The model under review builds one solid part; all positions refer to its coordinate system, in mm. Coordinates: 2 decimals unless noted, no trailing zeros. Write each loop counter-clockwise with the first axis right and the second up, starting at its lowest first coordinate (ties: lowest second). Pieces come first, ordered by that corner, then holes. Notation, with made-up numbers: (-25.75, -19) - (33.25, -19) arc R20 cw to (33.25, 0) - close; hole circle Ø5 at (-24, 76.25). An arc over 180 degrees is marked (long way). Return JSON: item names as keys, results as strings. Group by question number.
(1) We need section B-B on z = 159. State the section outline as (x, y) points, then the cut area to 3 significant figures.
(2) To check wall thickness, follow L1, parallel to X at y = -10, z = 160.5; L2, parallel to Z at x = 140.8, y = -4.75; L3, parallel to Z at x = 100.8, y = -5.5. State the ranges of each line that lie inside material, in increasing order. Write a range as from..to.
(3) We need section D-D on y = -6. State the section outline as (x, z) points (3 decimals).
(4) For pin 1 Ø11.5 at (x, z) = (180.8, 160) entering from +Y, flat-tipped, find the tip position at first contact; note if it passes through.
(5) We need section C-C on x = 140.8. State the section outline as (y, z) points.
(6) Draft analysis for pull direction X (two halves, no side actions). For faces 1 (the face through (90, -6, 145)), 2 (the face through (142, -12.7, 140)), 3 (the face through (100, -6.3, 166.3)), 4 (the face through (191.6, -6, 146)), state which applies: released by +X, released by -X, zero draft, split by the parting line, or undercut.
(7) We need section A-A on x = 100.8. State the section outline as (y, z) points, then the cut area to 3 significant figures.
```python
from build123d import *

# Parameters (mm, degrees)
SKETCH057_R  = 3.571875
PAD057_DEPTH = 30
SKETCH056_R  = 6.35
PAD056_DEPTH = 12.7


with BuildPart() as body056:
    # Sketch057 → Pad057 (new body)
    with BuildSketch(Plane.XZ):
        Circle(SKETCH057_R)
    extrude(amount=PAD057_DEPTH)


with BuildPart() as body056_1:
    # Body056 placement: moved
    add(body056.part.moved(Location((41.6, 2, 149.369))))


with BuildPart() as cut048:
    # Sketch056 → Pad056 (new body)
    with BuildSketch(Plane.XZ):
        with BuildLine():
            Line((-50.8, 110), (-50.8, 160.8))
            Line((-50.8, 160.8), (50.8, 160.8))
            Line((50.8, 160.8), (50.8, 110))
            Line((50.8, 110), (13.325, 110))
            ThreePointArc((13.325, 110), (0, 123.324965), (-13.325, 110))
            Line((-50.8, 110), (-13.325, 110))
        make_face()
        with Locations((-40, 150)):
            Circle(SKETCH056_R, mode=Mode.SUBTRACT)
        with Locations((40, 150)):
            Circle(SKETCH056_R, mode=Mode.SUBTRACT)
    extrude(amount=PAD056_DEPTH)


with BuildPart() as cut048_1:
    # Body057 placement: moved
    add(cut048.part.moved(Location((41.6, 0, 10))))

    # Cut048: cut Body056
    add(body056_1.part, mode=Mode.SUBTRACT)


with BuildPart() as cut048_2:
    # Cut048 placement: moved
    add(cut048_1.part.moved(Location((99.2, 0, 0))))


solid = cut048_2.part
```
Ans:
{
 "1": {"outline": "(90, -12.7) - (94.53, -12.7) - (94.53, 0) - (90, 0) - close; (107.07, -12.7) - (174.53, -12.7) - (174.53, 0) - (107.07, 0) - close; (187.07, -12.7) - (191.6, -12.7) - (191.6, 0) - (187.07, 0) - close", "area": "972 mm²"},
 "2": {"L1": "90..94.47, 107.13..174.47, 187.13..191.6", "L2": "133.32..145.8, 152.94..170.8", "L3": "120..153.65, 166.35..170.8"},
 "3": {"outline": "(90, 120) - (127.475, 120) arc R13.325 cw to (154.125, 120) - (191.6, 120) - (191.6, 170.8) - (90, 170.8) - close; hole circle Ø12.7 at (100.8, 160); hole circle Ø7.144 at (140.8, 149.369); hole circle Ø12.7 at (180.8, 160)"},
 "4": {"pin 1": "through"},
 "5": {"outline": "(-12.7, 133.32) - (0, 133.32) - (0, 145.8) - (-12.7, 145.8) - close; (-12.7, 152.94) - (0, 152.94) - (0, 170.8) - (-12.7, 170.8) - close"},
 "6": {"face 1": "released by -X", "face 2": "zero draft", "face 3": "undercut", "face 4": "released by +X"},
 "7": {"outline": "(-12.7, 120) - (0, 120) - (0, 153.65) - (-12.7, 153.65) - close; (-12.7, 166.35) - (0, 166.35) - (0, 170.8) - (-12.7, 170.8) - close", "area": "484 mm²"}
}
